Could you check a few things on this model? Use its own coordinates, in mm. A direction names the side the tool comes from. Coordinates: 2 decimals unless noted, no trailing zeros. Write each loop counter-clockwise with the first axis right and the second up, starting at its lowest first coordinate (ties: lowest second). Pieces come first, ordered by that corner, then holes.
Item 1: I want a section at B-B on y = -6.5. Please give me the cut outline in (x, z), then the cut area to 3 significant figures.
Item 2: For P1, Ø6, axis at x = 14.5, z = -12.5, coming from the +Y side; P2, Ø10, axis at y = 26, z = -7.5, coming from the -X side; P3, Ø3.5, axis at x = 0.5, y = 26.5, coming from the +Z side, each with a flat end and sliding along its axis, tell me the tip position at first contact or that it passes through.
Item 3: I want a section at C-C on x = -19.5. Please give me the cut outline in (y, z).
Item 4: I want a section at D-D on z = -3.5. Please give me the cut outline in (x, y), then the cut area to 3 significant figures.
Item 5: If I drill on probe 1 along X at (y, z) = (-0.5, -6.5); probe 2 along Z at (x, y) = (0.5, 28.5); probe 3 along X at (y, z) = (-26.5, -10), over which ranges is the centre line in solid material (lowest first)?
Item 6: I want a section at A-A on z = -15.25. State how many separate pieces and enclosed holes the cut face has, then the cut area to 3 significant figures.
Item 7: Which directions (+Z, -Z, +X, -X, +Y, -Y) give clear straight access to the entire face, cutting with the end or side of a thin tool? Please do faces 1 (the cylindrical face through (18.434, 28.913, -12.629)), 2 (the flat face through (0, -23, -0.762)), 3 (the flat face through (-19, 19, -17.78)).
Item 8: Thinking about a two-plate mould opening in X: for faces 4 (the flat face through (15, 0, -17.78)), 5 (the flat face through (-1.88, -16.34, -12.63)), which applies, +X half, -X half, draft (parallel to the pull), parting line (faces both ways), or undercut?
from build123d import *

# Parameters (mm, degrees)
F0_R            = 38.1
F0_R_2          = 34.29
F1_DEPTH        = 7.62
F2_DEPTH        = 17.78
F4_DEPTH        = 10.16
F5_DEPTH        = 10.16
F5_COPIES_COUNT = 4
F6_DEPTH        = 10.16
F6_COPIES_COUNT = 8
F8_DEPTH        = 0.762


# Not quite as in the source:
# - a pattern or mirror of a feature is missing from the dataset's text; its kind, count and spacing are read off the source's solid


with BuildPart() as f1:
    # F0 (on Top) → F1 (new body)
    with BuildSketch(Plane.XY):
        Circle(F0_R)
        Circle(F0_R_2, mode=Mode.SUBTRACT)
        Circle(F0_R_2)
    extrude(amount=-F1_DEPTH)

    # F0 (on Top) → F2 (join)
    with BuildSketch(Plane.XY):
        Circle(F0_R)
        Circle(F0_R_2, mode=Mode.SUBTRACT)
    extrude(amount=-F2_DEPTH)

    # F3 (on face) → F4 (join)
    with BuildSketch(Plane(origin=(0, 0, -7.62), x_dir=(1, 0, 0), z_dir=(0, 0, -1))):
        with BuildLine():
            Line((-4.7088706862, -3.0087008594), (-0.9977636205, -2.3358227154))
            ThreePointArc((-0.9977636205, -2.3358227154), (0, -2.54), (0.9977636205, -2.3358227154))
            Line((0.9977636205, -2.3358227154), (4.7088706862, -3.0087008594))
            Line((4.7088706862, -3.0087008594), (2.5217636205, 0.3038227154))
            ThreePointArc((2.5217636205, 0.3038227154), (2.1997045256, 1.27), (1.524, 2.032))
            Line((1.524, 2.032), (0, 5.588))
            Line((0, 5.588), (-1.524, 2.032))
            ThreePointArc((-1.524, 2.032), (-2.1997045256, 1.27), (-2.5217636205, 0.3038227154))
            Line((-2.5217636205, 0.3038227154), (-4.7088706862, -3.0087008594))
        make_face()
    extrude(amount=F4_DEPTH)

    # F3 (on face) → F5 (join)
    with BuildSketch(Plane(origin=(0, 0, -7.62), x_dir=(1, 0, 0), z_dir=(0, 0, -1))):
        Polygon((3.81, 14.9225), (0, 17.7165), (-3.81, 14.9225), (0, 12.1285), align=None)
    f5 = extrude(amount=F5_DEPTH)

    # F5_copies: F5 ×4 about axis
    f5_copies_axis = Axis((0, 0, 0), (0, 0, 1))
    for i in range(1, F5_COPIES_COUNT):
        add(f5.rotate(f5_copies_axis, i * 360 / F5_COPIES_COUNT))

    # F3 (on face) → F6 (join)
    with BuildSketch(Plane(origin=(0, 0, -7.62), x_dir=(1, 0, 0), z_dir=(0, 0, -1))):
        Polygon((3.81, 26.7335), (0, 29.5275), (-3.81, 26.7335), (0, 23.9395), align=None)
    f6 = extrude(amount=F6_DEPTH)

    # F6_copies: F6 ×8 about axis
    f6_copies_axis = Axis((0, 0, 0), (0, 0, 1))
    for i in range(1, F6_COPIES_COUNT):
        add(f6.rotate(f6_copies_axis, i * 360 / F6_COPIES_COUNT))

    # F7 (on face) → F8 (cut)
    with BuildSketch(Plane.XY):
        with BuildLine():
            Line((-10.16, -10.16), (-10.16, -30.0805069771))
            ThreePointArc((-10.16, -30.0805069771), (0, -31.75), (10.16, -30.0805069771))
            Line((10.16, -30.0805069771), (10.16, -10.16))
            Line((10.16, -10.16), (0, -20.32))
            Line((0, -20.32), (-10.16, -10.16))
        make_face()
        with BuildLine():
            ThreePointArc((-25.4, 19.05), (-31.75, 0), (-25.4, -19.05))
            Line((-25.4, -19.05), (-25.4, 19.05))
        make_face()
        with BuildLine():
            ThreePointArc((25.4, -19.05), (31.75, 0), (25.4, 19.05))
            Line((25.4, 19.05), (25.4, -19.05))
        make_face()
        with BuildLine():
            ThreePointArc((9.8601311185, 30.1801311185), (0, 31.75), (-9.8601311185, 30.1801311185))
            Line((-9.8601311185, 30.1801311185), (0, 20.32))
            Line((0, 20.32), (9.8601311185, 30.1801311185))
        make_face()
    extrude(amount=-F8_DEPTH, mode=Mode.SUBTRACT)


solid = f1.part
Response values:
1. outline: (-37.54, -17.78) - (-33.67, -17.78) - (-33.67, -7.62) - (33.67, -7.62) - (33.67, -17.78) - (37.54, -17.78) - (37.54, 0) - (31.08, 0) - (31.08, -0.76) - (25.4, -0.76) - (25.4, 0) - (-25.4, 0) - (-25.4, -0.76) - (-31.08, -0.76) - (-31.08, 0) - (-37.54, 0) - close
1. area: 642 mm2
2. P1: stops at y = 36.32
2. P2: stops at x = -31.79
2. P3: stops at z = -0.76
3. outline: (-32.73, -17.78) - (-28.21, -17.78) - (-28.21, -7.62) - (-21.09, -7.62) - (-21.09, -17.78) - (-16.53, -17.78) - (-16.53, -7.62) - (16.53, -7.62) - (16.53, -17.78) - (21.09, -17.78) - (21.09, -7.62) - (28.21, -7.62) - (28.21, -17.78) - (32.73, -17.78) - (32.73, 0) - (-32.73, 0) - close
4. outline: circle Ø76.2 at (0, 0)
4. area: 4,560 mm2
5. probe 1: x = -38.1 to 38.1
5. probe 2: z = -17.78 to -0.76
5. probe 3: x = -27.37 to -21.76, -3.49 to 3.49, 21.76 to 27.37
6. separate pieces: 14
6. enclosed holes: 1
6. area: 1,160 mm2
7. face 1: -Z
7. face 2: +Z
7. face 3: -Z, +X, -X, +Y, -Y
8. face 4: draft
8. face 5: undercut
